Could you check a few things on this model? Use its own coordinates, in mm. A direction names the side the tool comes from. Coordinates: 2 decimals unless noted, no trailing zeros. Loops run counter-clockwise (first coordinate to the right, second up) from the corner with the lowest first, then second, coordinate; pieces in that order, holes last. Notation, with made-up numbers: M 3.25,-28.5 L 18.25,-28.5 A17 cw 18.25,-17.5 Z; hole C -14,77.25 d3. An arc over 180 degrees is marked long. Write each question's results on one line, items separated by ' | '.
```python
from build123d import *

# Parameters (mm, degrees)
F1_DEPTH = 3.5


with BuildPart() as f1:
    # F0 (on Top) → F1 (new body)
    with BuildSketch(Plane.XY):
        with BuildLine():
            ThreePointArc((0.7, 1.658312), (0, -1.8), (-0.7, 1.658312))
            Line((-0.7, 1.658312), (-0.7, 10.245279))
            ThreePointArc((-0.7, 10.245279), (-1.63423, 9.524729), (-1.999757, 8.402958))
            Line((-1.999757, 8.402958), (-1.999757, 8.340602))
            Line((-1.999757, 8.340602), (-1.999757, 7.5))
            Line((-1.999757, 7.5), (-1.8, 7.5))
            Line((-1.8, 7.5), (-1.8, 3))
            Line((-1.8, 3), (-3.3, 3))
            Line((-3.3, 3), (-3.3, 0))
            ThreePointArc((-3.3, 0), (0, -3.3), (3.3, 0))
            Line((3.3, 0), (3.3, 3))
            Line((3.3, 3), (1.8, 3))
            Line((1.8, 3), (1.8, 7.5))
            Line((1.8, 7.5), (1.999125, 7.5))
            Line((1.999125, 7.5), (1.999125, 8.312613))
            Line((1.999125, 8.312613), (1.999125, 8.430947))
            ThreePointArc((1.999125, 8.430947), (1.626121, 9.536138), (0.7, 10.245279))
            Line((0.7, 10.245279), (0.7, 1.658312))
        make_face()
        with BuildLine():
            Line((-1.999757, 8.340602), (-1.999757, 8.402958))
            ThreePointArc((-1.999757, 8.402958), (-2, 8.37178), (-1.999757, 8.340602))
        make_face()
        with BuildLine():
            ThreePointArc((1.999125, 8.312613), (2, 8.37178), (1.999125, 8.430947))
            Line((1.999125, 8.430947), (1.999125, 8.312613))
        make_face()
    extrude(amount=F1_DEPTH)


solid = f1.part
```
(1) Imagine slicing it at D-D, the plane y = -0.5. List the corners of the cut face in (x, z) for me, and give its area (3 significant figures).
Reported:
outline: M -3.26,0 L -1.73,0 L -1.73,3.5 L -3.26,3.5 Z; M 1.73,0 L 3.26,0 L 3.26,3.5 L 1.73,3.5 Z | area: 10.7 mm2
(2) Imagine slicing it at B-B, the plane y = 2. List the corners of the cut face in (x, z) for me.
Reported:
outline: M -3.3,0 L -0.7,0 L -0.7,3.5 L -3.3,3.5 Z; M 0.7,0 L 3.3,0 L 3.3,3.5 L 0.7,3.5 Z
(3) Please list where these lines run through material, in increasing order: probe 1 along X at (y, z) = (0, 2.05); probe 2 along X at (y, z) = (3.5, 2.4); probe 3 along Y at (x, z) = (0, 1.1). Write a range as from..to.
Reported:
probe 1: x = -3.3..-1.8, 1.8..3.3 | probe 2: x = -1.8..-0.7, 0.7..1.8 | probe 3: y = -3.3..-1.8
(4) Will these pins go through, and if not, where does the flat tip stop? P1, Ø1, axis at y = 6.5, z = 1, coming from the -X side; P2, Ø1.5, axis at x = -2, z = 3, coming from the -Y side; P3, Ø0.7, axis at y = 8, z = 2.5, coming from the +X side; P4, Ø3, axis at x = -1, y = 1.5, coming from the -Z side.
Reported:
P1: stops at x = -1.8 | P2: stops at y = -3.05 | P3: stops at x = 2 | P4: stops at z = 0
(5) Which directions (+Z, -Z, +X, -X, +Y, -Y) give clear straight access to the entire face, cutting with the end or side of a thin tool? Please do faces 5 (the cylindrical face through (0.07, -1.8, 1.73)), 6 (the flat face through (1.999, 8, 2)), 7 (the flat face through (-2, 8, 2)), 8 (the flat face through (-3.3, 2, 2)), 9 (the flat face through (0.7, 6, 2)).
Reported:
face 5: +Z, -Z | face 6: +Z, -Z, +X, +Y | face 7: +Z, -Z, -X, +Y | face 8: +Z, -Z, -X, +Y, -Y | face 9: +Z, -Z, +Y
(6) If we mould it in two halves opening along Y, with no side actions, what happens to faces 1 (the flat face through (-0.7, 6, 2)), 2 (the flat face through (-1.8, 5, 2)), 3 (the flat face through (1.8, 5, 2)), 4 (the cylindrical face through (-0.1, -3.3, 1.7))? For each: released by +Y, released by -Y, zero draft, split by the parting line, or undercut.
Reported:
face 1: zero draft | face 2: undercut | face 3: undercut | face 4: released by -Y
(7) Imagine slicing it at A-A, the plane z = 1.6. List the corners of the cut face in (x, y) for me.
Reported:
outline: M -3.3,0 A3.3 ccw 3.3,0 L 3.3,3 L 1.8,3 L 1.8,7.5 L 2,7.5 L 2,8.31 A2 ccw 2,8.43 A2 ccw 0.7,10.25 L 0.7,1.66 A1.8 cw long -0.7,1.66 L -0.7,10.25 A2 ccw -2,8.4 A2 ccw -2,8.34 L -2,7.5 L -1.8,7.5 L -1.8,3 L -3.3,3 Z
(8) Imagine slicing it at C-C, the plane x = 0. List the corners of the cut face in (y, z) for me, and give its area (3 significant figures).
Reported:
outline: M -3.3,0 L -1.8,0 L -1.8,3.5 L -3.3,3.5 Z | area: 5.25 mm2
